Source: CAD feature listing. Evaluate the final solid. Frame: model axes, mm. A direction names the side the tool comes from. Give positions to 0.01 mm unless a question says otherwise; leave off trailing zeros. Loops run counter-clockwise (first coordinate to the right, second up) from the corner with the lowest first, then second, coordinate; pieces in that order, holes last. Notation, with made-up numbers: M -19.5,-31.5 L 35.5,-31.5 A27 cw 35.5,3.5 Z; hole C 28.25,83 d1. An arc over 180 degrees is marked long. Put each result on its own line as item: value.
from build123d import *

# Parameters (mm, degrees)
CUT_EXTRUDE1_DEPTH       = 57.404
SKETCH5_W                = 4.4958
SKETCH5_H                = 1.524
BOSS_EXTRUDE1_DEPTH      = 1.905
BOSS_EXTRUDE1_DEPTH_BACK = 52.705


with BuildPart() as part:
    # Sketch1 → Revolve2 (revolve)
    with BuildSketch(Plane.XY):
        with BuildLine():
            Line((0, 25.4), (0, 1.524))
            Line((0, 1.524), (-3.175, 1.524))
            ThreePointArc((-3.175, 1.524), (-3.624012806, 1.338012806), (-3.81, 0.889))
            Line((-3.81, 0.889), (-3.81, 0.635))
            ThreePointArc((-3.81, 0.635), (-3.624012806, 0.185987194), (-3.175, 0))
            Line((-3.175, 0), (0, 0))
            Line((0, 0), (0, -7.62))
            Line((0, -7.62), (25.4, -7.62))
            Line((25.4, -7.62), (25.4, 25.4))
            Line((25.4, 25.4), (0, 25.4))
        make_face()
    revolve(axis=Axis((25.4, -7.62, 0), (0, 1, 0)))

    # Sketch4 → Cut-Extrude1 (cut)
    with BuildSketch(Plane(origin=(0.035154624, -7.62, 1.335896343), x_dir=(0.052594344, 0, 0.99861596), z_dir=(-0.99861596, 0, 0.052594344))):
        with BuildLine():
            Line((-23.495, 9.144), (-26.67, 9.144))
            Line((-26.67, 9.144), (-26.67, 33.02))
            Line((-26.67, 33.02), (-24.13, 33.02))
            ThreePointArc((-24.13, 33.02), (-22.333948776, 32.276051224), (-21.59, 30.48))
            Line((-21.59, 30.48), (-21.59, 11.049))
            ThreePointArc((-21.59, 11.049), (-22.147961582, 9.701961582), (-23.495, 9.144))
        make_face()
        with BuildLine():
            Line((21.59, 30.48), (21.59, 11.049))
            ThreePointArc((21.59, 11.049), (22.147961582, 9.701961582), (23.495, 9.144))
            Line((23.495, 9.144), (26.67, 9.144))
            Line((26.67, 9.144), (26.67, 33.02))
            Line((26.67, 33.02), (24.13, 33.02))
            ThreePointArc((24.13, 33.02), (22.333948776, 32.276051224), (21.59, 30.48))
        make_face()
    extrude(amount=-CUT_EXTRUDE1_DEPTH, mode=Mode.SUBTRACT)

    # Sketch5 → Boss-Extrude1 (add, two sides)
    with BuildSketch(Plane(origin=(26.735896343, 0, 25.364845376), x_dir=(0.99861596, 0, -0.052594344), z_dir=(0.052594344, 0, 0.99861596))) as boss_extrude1_sk:
        with Locations((0, -6.858)):
            Rectangle(SKETCH5_W, SKETCH5_H)
    extrude(amount=BOSS_EXTRUDE1_DEPTH)
    extrude(boss_extrude1_sk.sketch, amount=-BOSS_EXTRUDE1_DEPTH_BACK)


solid = part.part
1. Contact query for flat-ended pins moving along their axis: P1, Ø0.7, axis at x = 25, z = -26.5, coming from the +Y side; P2, Ø3, axis at x = 13, y = 5, coming from the -Z side; P3, Ø1.5, axis at y = 3, z = -11, coming from the +X side. Output: stop coordinate, or through.
Found:
P1: y = 1.52
P2: z = -21.05
P3: x = 48.64
2. Access query for faces 1 (the cylindrical face through (24.05, 2.1, -22.09)), 2 (the flat face through (24.54, -6.87, 26.4)), 3 (the flat face through (29.03, -6.87, 26.16)), 4 (the flat face through (23.932, -6.847, -27.266)), 5 (the cylindrical face through (26.38, 2.1, 22.11)). Directions: +Z, -Z, +X, -X, +Y, -Y. A direction counts if a zero-diameter tool reaches every point of the face in a straight line with its end or side. Return the directions, or none.
Found:
face 1: -Z, -X
face 2: +Z, -X, -Y
face 3: +X, -Y
face 4: -Z, -X, -Y
face 5: +Z, +X
3. Section query C-C (y = 10.5). Output: boundary loops of the cut face in (x, z), plus the area to 3 significant figures.
Found:
outline: M 10.9,-20.86 L 37.63,-22.26 A25.4 ccw 39.9,20.86 L 13.17,22.26 A25.4 ccw Z
area: 1,890 mm^2
4. Section query A-A (z = 0). Output: boundary loops of the cut face in (x, y) (3 decimals), plus the area to 3 significant figures.
Found:
outline: M -3.81,0.635 A0.635 ccw -3.175,0 L 0,0 L 0,-7.62 L 50.8,-7.62 L 50.8,0 L 53.975,0 A0.635 ccw 54.61,0.635 L 54.61,0.889 A0.635 ccw 53.975,1.524 L 50.8,1.524 L 50.8,25.4 L 0,25.4 L 0,1.524 L -3.175,1.524 A0.635 ccw -3.81,0.889 Z
area: 1,690 mm^2
5. Section query B-B (y = -3). Output: boundary loops of the cut face in (x, z).
Found:
outline: C 25.4,0 d50.8
6. Material intervals for line 1 (Y direction, x = 0, z = -8); line 2 (X direction, y = 22, z = -11.5); line 3 (Z direction, x = 16.5, y = 16), sorted ascending. Write a range as from..to.
Found:
line 1: 0..1.52
line 2: 2.75..48.05
line 3: -21.15..22.09
